from build123d import *

# Parameters (mm, degrees)
F0_R     = 88.9
F1_DEPTH = 25.4
F2_D     = 20.6375
F4_D     = 50.8


# Not quite as in the source:
# - a feature names something its author has since deleted; it is built from what else it names


with BuildPart() as f1:
    # F0 (on Top) → F1 (new body)
    with BuildSketch(Plane.XY):
        Circle(F0_R)
    extrude(amount=F1_DEPTH)

    # F2 (through all)
    with Locations(Plane(origin=(0, 0, 0), x_dir=(1, 0, 0), z_dir=(0, 0, -1))):
        with Locations((0, -63.5), (-44.9012806053, -44.9012806053), (-63.5, 0), (-44.9012806053, 44.9012806053), (44.9012806053, 44.9012806053), (0, 63.5), (63.5, 0), (44.9012806053, -44.9012806053)):
            Hole(F2_D / 2)

    # F4 (through all)
    with Locations(Plane.XY.offset(25.4)):
        with Locations((0, 0)):
            Hole(F4_D / 2)


solid = f1.part
Geometry: final body of the model. Coordinates: model frame, mm. Round coordinates to 2 decimals unless told otherwise and drop trailing zeros. Order: outer loops, then holes, each group sorted by start corner. A loop starts at its lowest first (then second) coordinate and runs counter-clockwise, first axis right, second up. Notation, with made-up numbers: (10.5, 48) - (31.5, 48) arc R31 ccw to (31.5, 75) - close; hole circle Ø10 at (54, 18). An arc over 180 degrees is marked (long way). Write each question's results on one line, items separated by ' | '.
Item 1: First-contact query: pin 1 Ø5 at (x, z) = (7.5, 12.5) entering from +Y; pin 2 Ø2 at (y, z) = (12.5, 19) entering from -X; pin 3 Ø1.5 at (y, z) = (-50.5, 21) entering from +X. Flat tips, straight axial feed; report the tip coordinate or a pass-through.
Completed:
pin 1: y = 88.76 | pin 2: x = -88.15 | pin 3: x = 73.68
Item 2: Section C-C, the plane x = 63.5. Return the cut outline in (y, z).
Completed:
outline: (-62.22, 0) - (-10.32, 0) - (-10.32, 25.4) - (-62.22, 25.4) - close; (10.32, 0) - (62.22, 0) - (62.22, 25.4) - (10.32, 25.4) - close
Item 3: Section B-B, the plane x = -6. Return the cut outline in (y, z).
Completed:
outline: (-88.7, 0) - (-71.9, 0) - (-71.9, 25.4) - (-88.7, 25.4) - close; (-55.1, 0) - (-24.68, 0) - (-24.68, 25.4) - (-55.1, 25.4) - close; (24.68, 0) - (55.1, 0) - (55.1, 25.4) - (24.68, 25.4) - close; (71.9, 0) - (88.7, 0) - (88.7, 25.4) - (71.9, 25.4) - close
Item 4: Section A-A, the plane y = 0. Return the cut outline in (x, z).
Completed:
outline: (-88.9, 0) - (-73.82, 0) - (-73.82, 25.4) - (-88.9, 25.4) - close; (-53.18, 0) - (-25.4, 0) - (-25.4, 25.4) - (-53.18, 25.4) - close; (25.4, 0) - (53.18, 0) - (53.18, 25.4) - (25.4, 25.4) - close; (73.82, 0) - (88.9, 0) - (88.9, 25.4) - (73.82, 25.4) - close
Item 5: Material intervals for line 1 along Y through (x, z) = (0, 8); line 2 along X through (y, z) = (7, 14); line 3 along Y through (x, z) = (46, 20), sorted ascending. Write a range as [from, to].
Completed:
line 1: [-88.9, -73.82], [-53.18, -25.4], [25.4, 53.18], [73.82, 88.9] | line 2: [-88.62, -71.08], [-55.92, -24.42], [24.42, 55.92], [71.08, 88.62] | line 3: [-76.07, -55.16], [-34.64, 34.64], [55.16, 76.07]
Item 6: Mould query, pull axis Y, two halves, no side actions, for faces 1 (the cylindrical face through (84.795, 26.703, 12.522)), 2 (the flat face through (19, -19, 0)), 3 (the cylindrical face through (1.34, -73.73, 12.88)). Classes: pulls with the +Y half, pulls with the -Y half, needs draft (parallel to the pull), parting line crosses it, or undercut.
Completed:
face 1: parting line crosses it | face 2: needs draft | face 3: undercut
